Geometry: final body of the model. Coordinates: model frame, mm. A direction names the side the tool comes from. Coordinates: 2 decimals unless noted, no trailing zeros. Order: outer loops, then holes, each group sorted by start corner. A loop starts at its lowest first (then second) coordinate and runs counter-clockwise, first axis right, second up. Notation, with made-up numbers: (82, -18) - (139, -18) arc R10 ccw to (139, -5) - close; hole circle Ø2 at (21, -10.5). An arc over 180 degrees is marked (long way). Use a Markdown table: item, result. Add a question column.
```python
from build123d import *

# Parameters (mm, degrees)
ESQUISSE1_W                  = 28
ESQUISSE1_H                  = 20
BOSS_EXTRU_1_DEPTH           = 2
ESQUISSE2_W                  = 2
ESQUISSE2_H                  = 20
BOSS_EXTRU_2_DEPTH           = 10
ENL_V_MAT_EXTRU_1_DEPTH      = 22.354156504
ENL_V_MAT_EXTRU_1_DEPTH_BACK = 22.354156504
ESQUISSE3_R                  = 1.5


with BuildPart() as part:
    # Esquisse1 → Boss.-Extru.1 (new body)
    with BuildSketch(Plane.XY):
        Rectangle(ESQUISSE1_W, ESQUISSE1_H)
    extrude(amount=BOSS_EXTRU_1_DEPTH)

    # Esquisse2 → Boss.-Extru.2 (add)
    with BuildSketch(Plane.XY):
        with Locations((-15, 0)):
            Rectangle(ESQUISSE2_W, ESQUISSE2_H)
        with Locations((15, 0)):
            Rectangle(ESQUISSE2_W, ESQUISSE2_H)
    extrude(amount=BOSS_EXTRU_2_DEPTH)

    # Esquisse3 → Enlèv. mat.-Extru.1 (cut, two sides: drawn at the far end of the back side and taken through both)
    with BuildSketch(Plane(origin=(0, 0, 0), x_dir=(0, 0, -1), z_dir=(1, 0, 0)).offset(-ENL_V_MAT_EXTRU_1_DEPTH_BACK)):
        with Locations((-5, 0)):
            Circle(ESQUISSE3_R)
    extrude(amount=ENL_V_MAT_EXTRU_1_DEPTH + ENL_V_MAT_EXTRU_1_DEPTH_BACK, mode=Mode.SUBTRACT)


solid = part.part
```
1) Section query D-D (y = 8.5). Return the cut outline in (x, z).
2) Draft query along Z for faces 1 (the flat face through (15, 0, 10)), 2 (the flat face through (-0.1, 10, 1.6)), 3 (the cylindrical face through (15, -0.9, 6.2)). Return one class per face: released by +Z, released by -Z, zero draft, split by the parting line, or undercut.
3) Line query: line 1 (X direction, y = 5.75, z = 6.5); line 2 (Y direction, x = -15.3, z = 5); line 3 (Z direction, x = 15.4, y = 0). Output: solid intervals per line, ascending. Write a range as from..to.
4) Access query for faces 4 (the flat face through (-14, 0, 7)), 5 (the flat face through (-16, 0, 3)). Directions: +Z, -Z, +X, -X, +Y, -Y. A direction counts if a zero-diameter tool reaches every point of the face in a straight line with its end or side. Return the directions, or none.
5) Section query B-B (z = 9). Return the cut outline in (x, y), and give its area (3 significant figures).
6) First-contact query: pin 1 (4 mm diameter, centred on x = -2, y = -7, fed in from +Z); pin 2 (4 mm diameter, centred on x = 11, z = 3.5, fed in from +Y). Flat tips, straight axial feed; report the tip coordinate or a pass-through.
7) Section query A-A (y = 0). Return the cut outline in (x, z).
8) Section query C-C (z = 5). Return the cut outline in (x, y), and give its area (3 significant figures).
From the geometry:
| question | item | result |
|---|---|---|
| 1 | outline | (-16, 0) - (16, 0) - (16, 10) - (14, 10) - (14, 2) - (-14, 2) - (-14, 10) - (-16, 10) - close |
| 2 | face 1 | released by +Z |
| 2 | face 2 | zero draft |
| 2 | face 3 | undercut |
| 3 | line 1 | x = -16..-14, 14..16 |
| 3 | line 2 | y = -10..-1.5, 1.5..10 |
| 3 | line 3 | z = 0..3.5, 6.5..10 |
| 4 | face 4 | +Z, +Y, -Y |
| 4 | face 5 | +Z, -Z, -X, +Y, -Y |
| 5 | outline | (-16, -10) - (-14, -10) - (-14, 10) - (-16, 10) - close; (14, -10) - (16, -10) - (16, 10) - (14, 10) - close |
| 5 | area | 80.0 mm^2 |
| 6 | pin 1 | stops at z = 2 |
| 6 | pin 2 | stops at y = 10 |
| 7 | outline | (-16, 0) - (16, 0) - (16, 3.5) - (14, 3.5) - (14, 2) - (-14, 2) - (-14, 3.5) - (-16, 3.5) - close; (-16, 6.5) - (-14, 6.5) - (-14, 10) - (-16, 10) - close; (14, 6.5) - (16, 6.5) - (16, 10) - (14, 10) - close |
| 8 | outline | (-16, -10) - (-14, -10) - (-14, -1.5) - (-16, -1.5) - close; (-16, 1.5) - (-14, 1.5) - (-14, 10) - (-16, 10) - close; (14, -10) - (16, -10) - (16, -1.5) - (14, -1.5) - close; (14, 1.5) - (16, 1.5) - (16, 10) - (14, 10) - close |
| 8 | area | 68.0 mm^2 |
